Here's how the part is built. I have some questions about the finished solid (model axes, mm). A direction names the side the tool comes from. Coordinates: 2 decimals unless noted, no trailing zeros. Loops run counter-clockwise (first coordinate to the right, second up) from the corner with the lowest first, then second, coordinate; pieces in that order, holes last. Notation, with made-up numbers: (58, -33.75) -> (115, -33.75) arc R19 cw to (115, -4.75) -> close; hole circle Ø2 at (2, 48.25). An arc over 180 degrees is marked (long way). Answer as a JSON object with one key per item and string values. Group by question number.
1) If we mould it in two halves opening along X, with no side actions, what happens to faces 1 (the flat face through (-14, 6.5, 2.5)), 2 (the flat face through (-37.5, 6.5, -0.2)), 3 (the flat face through (-4, 6.5, 6.5))? For each: +X half, -X half, draft (parallel to the pull), parting line (faces both ways), or undercut.
2) I want a section at C-C (z = 0). Count the separate pieces of the cut face and the enclosed holes in it, then the cut area to 3 significant figures.
3) I want a section at D-D (x = -18.5). Write out the boundary of the cut face in (y, z).
4) I want a section at A-A (x = -26.5). Write out the boundary of the cut face in (y, z), then the cut area to 3 significant figures.
5) I'm going to push flat-ended pins straight in: pin 1 (2 mm diameter, centred on y = -9, z = -7, fed in from +X); pin 2 (3 mm diameter, centred on y = -6.5, z = 5, fed in from +X); pin 3 (6 mm diameter, centred on x = -5.5, z = -3.5, fed in from -Y). Where does each tip first touch, or does it pass through?
6) Which directions (+Z, -Z, +X, -X, +Y, -Y) give clear straight access to the entire face, cutting with the end or side of a thin tool? Please do faces 4 (the flat face through (-18.2, 6.5, -10.5)), 5 (the conical face through (-34.21, -20.49, 10.19)), 6 (the flat face through (-30, -7, -10)).
7) I need wall thicknesses on probe 1 along Y at (x, z) = (-35.65, 0); probe 2 along X at (y, z) = (-7.25, -9.25); probe 3 along X at (y, z) = (-10, -7.75). Which ranges of each line are inside material? Lowest first, please. Write a range as [from, to].
```python
from build123d import *

# Parameters (mm, degrees)
CROQUIS1_R              = 2.1
SALIENTE_EXTRUIR1_DEPTH = 7
CROQUIS2_W              = 28
CROQUIS2_H              = 28
CROQUIS2_W_2            = 20
CROQUIS2_H_2            = 20
SALIENTE_EXTRUIR2_DEPTH = 28
CROQUIS3_W              = 6
CROQUIS3_H              = 1
CROQUIS3_W_2            = 1
CROQUIS3_H_2            = 6
SALIENTE_EXTRUIR3_DEPTH = 28
REDONDEO1_R             = 0.5
REDONDEO2_R             = 2
REDONDEO3_R             = 2
CHAFL_N1_SIZE           = 1
CHAFL_N3_SIZE           = 1
CORTAR_EXTRUIR2_REACH   = 53.595
CROQUIS4_R              = 2.1


with BuildPart() as part:
    # Croquis1 → Saliente-Extruir1 (new, symmetric)
    with BuildSketch(Plane(origin=(0, 0, 0), x_dir=(1, 0, 0), z_dir=(0, 1, 0))):
        with BuildLine():
            Line((0, 7), (-10, 7))
            Line((-10, 7), (-10, -6.999720999))
            Line((-10, -6.999720999), (0.062497509, -6.999720999))
            ThreePointArc((0.062497509, -6.999720999), (6.999930249, 0.031249066), (0, 7))
        make_face()
        with Locations(Location((0, 0, 0), (0, 0, 270))):
            Circle(CROQUIS1_R, mode=Mode.SUBTRACT)
    extrude(amount=SALIENTE_EXTRUIR1_DEPTH, both=True)

    # Croquis2 → Saliente-Extruir2 (add)
    with BuildSketch(Plane(origin=(0, 7, 0), x_dir=(1, 0, 0), z_dir=(0, 1, 0))):
        with Locations((-24, 0)):
            Rectangle(CROQUIS2_W, CROQUIS2_H)
        with Locations((-24, 0)):
            Rectangle(CROQUIS2_W_2, CROQUIS2_H_2, mode=Mode.SUBTRACT)
    extrude(amount=-SALIENTE_EXTRUIR2_DEPTH)

    # Croquis3 → Saliente-Extruir3 (add, through all)
    with BuildSketch(Plane(origin=(0, 7, 0), x_dir=(1, 0, 0), z_dir=(0, 1, 0))):
        with Locations((-24, 9.5)):
            Rectangle(CROQUIS3_W, CROQUIS3_H)
        with Locations((-14.5, 0)):
            Rectangle(CROQUIS3_W_2, CROQUIS3_H_2)
        with Locations((-24, -9.5)):
            Rectangle(CROQUIS3_W, CROQUIS3_H)
        with Locations((-33.5, 0)):
            Rectangle(CROQUIS3_W_2, CROQUIS3_H_2)
    extrude(amount=-SALIENTE_EXTRUIR3_DEPTH)

    # Redondeo1
    redondeo1_edges = [part.edges().sort_by_distance(p)[0] for p in [
        (-14, -7, 10),
        (-34, -7, 10),
        (-34, -7, -10),
        (-14, -7, -10),
    ]]
    fillet(redondeo1_edges, radius=REDONDEO1_R)

    # Redondeo2
    redondeo2_edges = [part.edges().sort_by_distance(p)[0] for p in [
        (-10, -7, -14),
        (-10, -7, 14),
        (-38, -7, 14),
        (-38, -7, -14),
    ]]
    fillet(redondeo2_edges, radius=REDONDEO2_R)

    # Redondeo3
    redondeo3_edges = [part.edges().sort_by_distance(p)[0] for p in [
        (-10, 0, 6.999720999),
        (-10, 0, -7),
    ]]
    fillet(redondeo3_edges, radius=REDONDEO3_R)

    # Chaflán1
    chafl_n1_edges = [part.edges().sort_by_distance(p)[0] for p in [
        (-30.25, -21, 10),
        (-14.146446609, -21, 9.853553391),
        (-14.146446609, -21, -9.853553391),
        (-33.853553391, -21, -9.853553391),
        (-33.853553391, -21, 9.853553391),
        (-24, -21, -14),
        (-38, -21, 0),
        (-10, -21, 0),
        (-24, -21, 14),
        (-10.585786438, -21, 13.414213562),
        (-37.414213562, -21, 13.414213562),
        (-10.585786438, -21, -13.414213562),
        (-37.414213562, -21, -13.414213562),
        (-30.25, -21, -10),
        (-21, -21, -9.5),
        (-24, -21, -9),
        (-27, -21, -9.5),
        (-14, -21, -6.25),
        (-14.5, -21, 3),
        (-15, -21, 0),
        (-14.5, -21, -3),
        (-17.75, -21, 10),
        (-27, -21, 9.5),
        (-24, -21, 9),
        (-21, -21, 9.5),
        (-34, -21, 6.25),
        (-33, -21, 0),
        (-33.5, -21, 3),
        (-33.5, -21, -3),
        (-14, -21, 6.25),
        (-17.75, -21, -10),
        (-34, -21, -6.25),
    ]]
    chamfer(chafl_n1_edges, length=CHAFL_N1_SIZE)

    # Chaflán3
    chafl_n3_edges = [part.edges().sort_by_distance(p)[0] for p in [
        (-21, 7, -9.5),
        (-24, 7, -9),
        (-27, 7, -9.5),
        (-30.25, 7, -10),
        (-33.853553391, 7, -9.853553391),
        (-34, 7, -6.25),
        (-33.5, 7, -3),
        (-33, 7, 0),
        (-33.5, 7, 3),
        (-34, 7, 6.25),
        (-33.853553391, 7, 9.853553391),
        (-30.25, 7, 10),
        (-27, 7, 9.5),
        (-24, 7, 9),
        (-21, 7, 9.5),
        (-17.75, 7, 10),
        (-14.146446609, 7, 9.853553391),
        (-14, 7, 6.25),
        (-14.5, 7, 3),
        (-15, 7, 0),
        (-14.5, 7, -3),
        (-14, 7, -6.25),
        (-14.146446609, 7, -9.853553391),
        (-17.75, 7, -10),
        (0, 7, -2.1),
        (-10.585786438, 7, -13.414213562),
        (-10, 7, -10.5),
        (-9.414213562, 7, -7.585786438),
        (-4, 7, -7),
        (6.999930249, 7, -0.031249066),
        (-3.968751246, 7, 6.999720999),
        (-9.414213562, 7, 7.585507436),
        (-10, 7, 10.499860499),
        (-10.585786438, 7, 13.414213562),
        (-24, 7, 14),
        (-37.414213562, 7, 13.414213562),
        (-38, 7, 0),
        (-37.414213562, 7, -13.414213562),
        (-24, 7, -14),
    ]]
    chamfer(chafl_n3_edges, length=CHAFL_N3_SIZE)

    # Croquis4 → Cortar-Extruir2 (cut, up to next)
    with BuildSketch(Plane.ZY.offset(38), mode=Mode.PRIVATE) as cortar_extruir2_sk1:
        Circle(CROQUIS4_R)
    cortar_extruir2_tool1 = extrude(cortar_extruir2_sk1.sketch, amount=-CORTAR_EXTRUIR2_REACH, mode=Mode.PRIVATE) & part.part
    # Croquis4 → Cortar-Extruir2 (cut, up to next)
    with BuildSketch(Plane.ZY.offset(38), mode=Mode.PRIVATE) as cortar_extruir2_sk2:
        with Locations((0, -14)):
            Circle(CROQUIS4_R)
    cortar_extruir2_tool2 = extrude(cortar_extruir2_sk2.sketch, amount=-CORTAR_EXTRUIR2_REACH, mode=Mode.PRIVATE) & part.part
    add(cortar_extruir2_tool1.solids().sort_by_distance((-38, 0, 0))[0], mode=Mode.SUBTRACT)
    add(cortar_extruir2_tool2.solids().sort_by_distance((-38, -14, 0))[0], mode=Mode.SUBTRACT)


solid = part.part
```
Determined:
{
 "1": {"face 1": "undercut", "face 2": "-X half", "face 3": "draft"},
 "2": {"separate pieces": "5", "enclosed holes": "0", "area": "412 mm^2"},
 "3": {"outline": "(-21, -13) -> (-20, -14) -> (6, -14) -> (7, -13) -> (7, -11) -> (6, -10) -> (-20, -10) -> (-21, -11) -> close; (-21, 11) -> (-20, 10) -> (6, 10) -> (7, 11) -> (7, 13) -> (6, 14) -> (-20, 14) -> (-21, 13) -> close"},
 "4": {"outline": "(-21, -13) -> (-20, -14) -> (6, -14) -> (7, -13) -> (7, -11) -> (6.5, -10.5) -> (6.5, -9.5) -> (6, -9) -> (-20, -9) -> (-20.5, -9.5) -> (-20.5, -10.5) -> (-21, -11) -> close; (-21, 11) -> (-20.5, 10.5) -> (-20.5, 9.5) -> (-20, 9) -> (6, 9) -> (6.5, 9.5) -> (6.5, 10.5) -> (7, 11) -> (7, 13) -> (6, 14) -> (-20, 14) -> (-21, 13) -> close", "area": "274 mm^2"},
 "5": {"pin 1": "x = -10", "pin 2": "x = 6.06", "pin 3": "y = -7"},
 "6": {"face 4": "+Y", "face 5": "-Y", "face 6": "+Y, -Y"},
 "7": {"probe 1": "[-21, -16.1], [-11.9, -2.1], [2.1, 7]", "probe 2": "[-38, -34], [-27, -21], [-14, -10]", "probe 3": "[-38, -34], [-14, -10]"}
}
